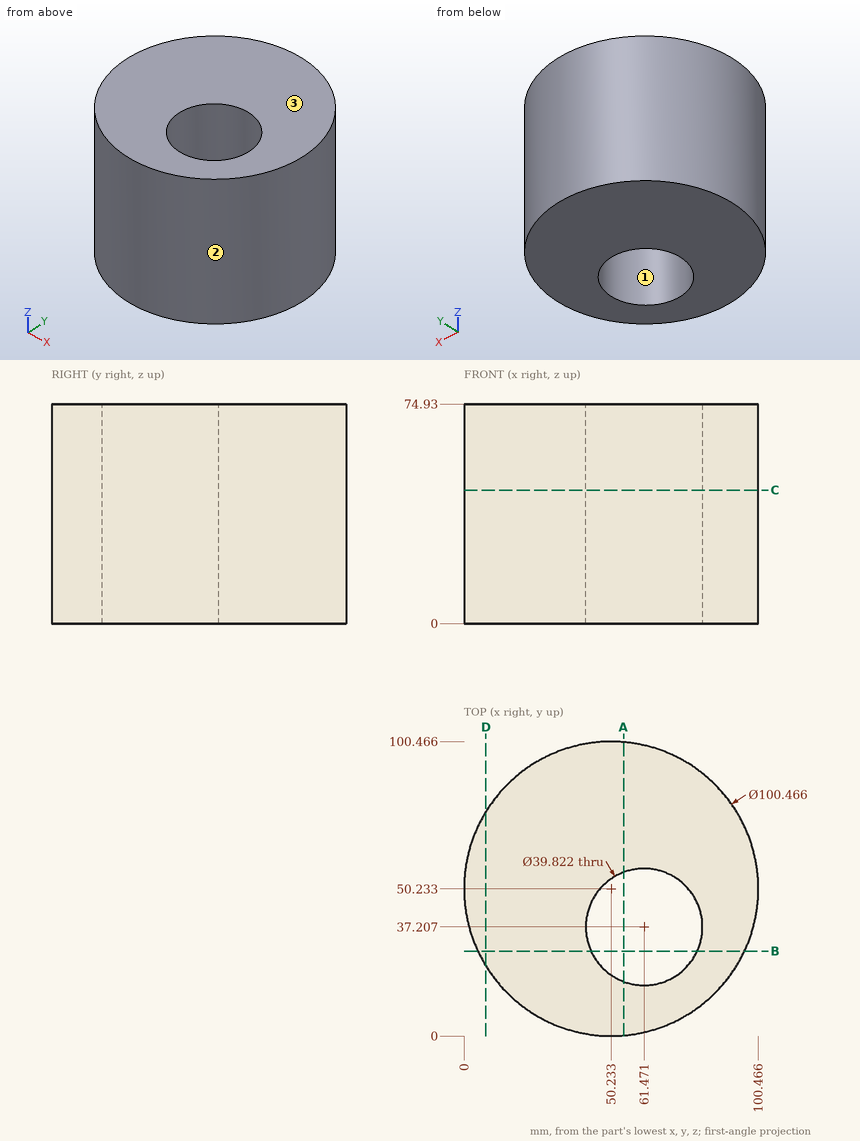
Geometry check sheet. Reference: drawing and pictorial views, mm from the part's lowest x, y, z. Round coordinates to 2 decimals unless told otherwise and drop trailing zeros. Write each loop counter-clockwise with the first axis right and the second up, starting at its lowest first coordinate (ties: lowest second). Pieces come first, ordered by that corner, then holes. Notation, with made-up numbers: (41.5, 72.5) -> (63.5, 72.5) arc R14 ccw to (63.5, 93.5) -> close; hole circle Ø4 at (79, -38). An arc over 180 degrees is marked (long way). Answer as CSV lines item,"result". Start each with the question number.
1) Release check for a two-part mould opening along X. For the marked faces 1, 2 and 3 record: pulls with the +X half, pulls with the -X half, needs draft (parallel to the pull), parting line crosses it, or undercut.
2) Go/stop test with flat-tipped pins: P1, Ø1, axis at y = 49.5, z = 29.5, coming from the -X side; P2, Ø6, axis at y = 43, z = 65, coming from the -X side; P3, Ø1, axis at y = 27.5, z = 66.5, coming from the -X side. Record where each tip stops, or that it passes through.
3) Section check B-B on y = 29. Enter the section's corners in (x, z), and give its area (3 significant figures).
4) Section check D-D on x = 7.5. Enter the section's corners in (y, z).
5) Section check C-C on z = 45.5. Enter the section's corners in (x, y), and give its area (3 significant figures).
6) Material ranges on line 1 (Y direction, x = 65, z = 36); line 2 (X direction, y = 51, z = 10) (1 decimal); line 3 (Y direction, x = 44.5, z = 13) (1 decimal), recorded low to high. Write a range as from..to.
7) Section check A-A on x = 54.5. Enter the section's corners in (y, z) (1 decimal).
Found:
1,face 1,"undercut"
1,face 2,"parting line crosses it"
1,face 3,"needs draft"
2,P1,"stops at x = 0"
2,P2,"stops at x = 0.18"
2,P3,"stops at x = 5.19"
3,outline,"(4.71, 0) -> (43.33, 0) -> (43.33, 74.93) -> (4.71, 74.93) -> close; (79.61, 0) -> (95.76, 0) -> (95.76, 74.93) -> (79.61, 74.93) -> close"
3,area,"4,100 mm^2"
4,outline,"(23.83, 0) -> (76.64, 0) -> (76.64, 74.93) -> (23.83, 74.93) -> close"
5,outline,"circle Ø100.47 at (50.23, 50.23); hole circle Ø39.82 at (61.47, 37.21)"
5,area,"6,680 mm^2"
6,line 1,"y = 2.22..17.61, 56.8..98.25"
6,line 2,"x = 0..47.1, 75.8..100.5"
6,line 3,"y = 0.3..26.8, 47.6..100.1"
7,outline,"(0.2, 0) -> (18.6, 0) -> (18.6, 74.9) -> (0.2, 74.9) -> close; (55.9, 0) -> (100.3, 0) -> (100.3, 74.9) -> (55.9, 74.9) -> close"
